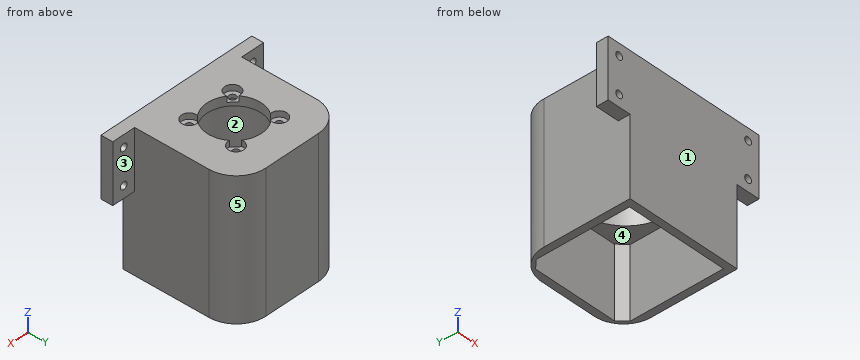
Autodesk Inventor part; units mm, degrees
ref_plane "YZ Plane" through (0, 0, 0) normal (1, 0, 0) x (0, 1, 0)
ref_plane "XZ Plane" through (0, 0, 0) normal (0, 1, 0) x (-1, 0, 0)
ref_plane "XY Plane" through (0, 0, 0) normal (0, 0, 1) x (1, 0, 0)
sketch "Sketch1" plane through (0, 0, 0) normal (0, 0, 1) x (1, 0, 0)
  line L0 (-21.5, -21.5) -> (21.5, -21.5)
  line L1 (21.5, -21.5) -> (21.5, 21.5)
  line L2 (21.5, 21.5) -> (-21.5, 21.5)
  line L3 (-21.5, 21.5) -> (-21.5, -21.5)
  line L4 (-21.5, -21.5) -> (21.5, 21.5) construction
  line L5 (21.5, -21.5) -> (-21.5, 21.5) construction
  circle A0 centre (0, 0) radius 18.5
  circle A1 centre (0, 0) radius 11.5
  circle A2 centre (0, 0) radius 14
  circle A3 centre (-9.8995, 9.8995) radius 1.5
  circle A4 centre (-9.8995, -9.8995) radius 1.5
  circle A5 centre (9.8995, -9.8995) radius 1.5
  circle A6 centre (9.8995, 9.8995) radius 1.5
  line L6 (0, 0) -> (0, 21.5)
  line L7 (-24.5, 24.5) -> (24.5, 24.5)
  line L8 (24.5, 24.5) -> (24.5, -24.5)
  line L9 (24.5, -24.5) -> (-24.5, -24.5)
  line L10 (-24.5, -24.5) -> (-24.5, 24.5)
  line L11 (-24.5, 24.5) -> (24.5, -24.5) construction
  line L12 (24.5, 24.5) -> (-24.5, -24.5) construction
  dimension "d4" = 28
  dimension "d0" = 43
  dimension "d1" = 43
  dimension "d2" = 37
  dimension "d3" = 23
  dimension "d5" = 3
  dimension "d8" = 360
  dimension "d10" = 3
  dimension "d11" = 3
extrude "Extrusion1" add sketch "Sketch1" along normal blind 5 and the other way blind 30 contours L7 L8 L9 L10
extrude "Extrusion2" add sketch "Sketch1" along normal blind 24 contours L3 L2 L1 L0
sketch "Sketch2" plane through (0, 0, 24) normal (0, 0, 1) x (1, 0, 0)
  circle A0 centre (0, 0) radius 11.5
  circle A1 centre (0, 0) radius 14
  circle A2 centre (9.8995, 9.8995) radius 1.5
  circle A3 centre (9.8995, -9.8995) radius 1.5
  circle A4 centre (-9.8995, -9.8995) radius 1.5
  circle A5 centre (-9.8995, 9.8995) radius 1.5
  circle A6 centre (0, 0) radius 18.5
  line L0 (-21.5, 21.5) -> (-21.5, -21.5)
  line L1 (-21.5, -21.5) -> (21.5, -21.5)
  line L2 (21.5, -21.5) -> (21.5, 21.5)
  line L3 (21.5, 21.5) -> (-21.5, 21.5)
  circle A7 centre (0, 0) radius 18.5
  line L4 (24.5, -24.5) -> (-24.5, -24.5)
  line L5 (24.5, 24.5) -> (24.5, -24.5)
  line L6 (-24.5, 24.5) -> (24.5, 24.5)
  line L7 (-24.5, -24.5) -> (-24.5, 24.5)
  line L8 (21.5, -21.5) -> (21.5, 21.5)
  line L9 (-21.5, -21.5) -> (21.5, -21.5)
  line L10 (-21.5, 21.5) -> (-21.5, -21.5)
  line L11 (21.5, 21.5) -> (-21.5, 21.5)
extrude "Extrusion3" add sketch "Sketch2" along normal blind 4 contours A1 A3 A4 A5 A2 | A6 | L3 L2 L1 L0
sketch "Sketch8" plane through (0, 0, 28) normal (0, 0, 1) x (1, 0, 0)
  line L0 (-24.5, -24.5) -> (24.5, -24.5)
  line L1 (24.5, -24.5) -> (24.5, 24.5)
  line L2 (24.5, 24.5) -> (-24.5, 24.5)
  line L3 (-24.5, 24.5) -> (-24.5, -24.5)
  line L4 (21.5, 21.5) -> (21.5, -21.5)
  line L5 (21.5, -21.5) -> (-21.5, -21.5)
  line L6 (-21.5, -21.5) -> (-21.5, 21.5)
  line L7 (-21.5, 21.5) -> (21.5, 21.5)
  line L8 (-21.5, 21.5) -> (-21.5, -21.5)
  line L9 (-21.5, -21.5) -> (21.5, -21.5)
  line L10 (21.5, -21.5) -> (21.5, 21.5)
  line L11 (21.5, 21.5) -> (-21.5, 21.5)
  circle A0 centre (-9.8995, 9.8995) radius 1.5
  circle A1 centre (-9.8995, -9.8995) radius 1.5
  circle A2 centre (9.8995, -9.8995) radius 1.5
  circle A3 centre (0, 0) radius 11.5
  circle A4 centre (9.8995, 9.8995) radius 1.5
extrude "Extrusion8" add sketch "Sketch8" against normal up to surface (23 mm away) contours L3 L2 L1 L0
sketch "Sketch9" plane through (-24.5, -24.5, -30) normal (0, -1, 0) x (1, 0, 0)
  line L0 (49, 0) -> (49, 58)
  line L1 (49, 58) -> (59, 58)
  line L2 (59, 58) -> (59, 33)
  line L3 (59, 33) -> (49, 33)
  line L4 (49, 33) -> (49, 58)
  line L5 (0, 58) -> (0, 0)
  line L6 (0, 58) -> (-10, 58)
  line L7 (-10, 58) -> (-10, 33)
  line L8 (-10, 33) -> (0, 33)
  line L9 (0, 33) -> (0, 58)
  line L10 (0, 58) -> (49, 58)
  circle A0 centre (54, 38) radius 1.55
  circle A1 centre (54, 53) radius 1.55
  circle A2 centre (-5, 38) radius 1.55
  circle A3 centre (-5, 53) radius 1.55
  point P0 (24.5, 30)
  point P1 (0, 33)
  point P2 (49, 33)
  dimension "d72" = 0
  dimension "d73" = 25
  dimension "d74" = 25
  dimension "d75" = 10
  dimension "d76" = 10
  dimension "d77" = 15
  dimension "d78" = 15
  dimension "d79" = 5
  dimension "d80" = 5
  dimension "d81" = 3.1
  dimension "d82" = 3.1
  dimension "d83" = 3.1
  dimension "d84" = 3.1
extrude "Extrusion9" add sketch "Sketch9" against normal blind 5
chamfer "Chamfer3" distance 3.5 angle 45 2 edges at (21.5, 21.5, -15) (-21.5, 21.5, -15)
fillet "Fillet10" radius 12.5 2 edges at (-24.5, 24.5, -1) (24.5, 24.5, -1)
sketch "Sketch10" plane through (0, 0, 28) normal (0, 0, 1) x (1, 0, 0)
  circle A0 centre (-9.8995, 9.8995) radius 1.5
  circle A1 centre (-9.8995, 9.8995) radius 3.25
  circle A2 centre (9.8995, 9.8995) radius 1.5
  circle A3 centre (9.8995, 9.8995) radius 3.25
  circle A4 centre (9.8995, -9.8995) radius 1.5
  circle A5 centre (9.8995, -9.8995) radius 3.25
  circle A6 centre (-9.8995, -9.8995) radius 1.5
  circle A7 centre (-9.8995, -9.8995) radius 3.25
  point P0 (0, 0)
  dimension "d94" = 6.5
  dimension "d95" = 6.5
  dimension "d96" = 6.5
  dimension "d97" = 6.5
extrude "Extrusion10" cut sketch "Sketch10" against normal blind 2.5 contours A0 | A1 | A2 | A3 | A4 | A5 | A6 | A7
properties part number "StepperMotorHolder"
For this review, take the finished solid that the model builds, in its own axes (mm). Face numbers are marked on the shaded views. A direction names the side the tool comes from. Round coordinates to 2 decimals unless told otherwise and drop trailing zeros. Write each loop counter-clockwise with the first axis right and the second up, starting at its lowest first coordinate (ties: lowest second). Pieces come first, ordered by that corner, then holes. Notation, with made-up numbers: (35.5, 26.25) -> (54.5, 26.25) arc R14 ccw to (54.5, 51.25) -> close; hole circle Ø1 at (29, -29). An arc over 180 degrees is marked (long way). Use one line per item in the form item = value.
1) Clearance check with flat-ended pins moving along their axes: pin 1 (3 mm diameter, centred on x = -16, y = 17.5, fed in from -Z); pin 2 (6 mm diameter, centred on y = -16, z = -13.5, fed in from -X); pin 3 (10 mm diameter, centred on y = 6, z = 20, fed in from +X). State where each tip first meets the part, or that it passes through.
Found:
pin_1 = 0
pin_2 = -24.5
pin_3 = 24.5
2) Tool access review of the marked faces 1 and 2: name each direction out of +Z, -Z, +X, -X, +Y, -Y from which nothing blocks a thin tool from reaching the whole face with its end or side.
Found:
face_1 = +Z, -Z, +X, -X, -Y
face_2 = -Z
3) To check wall thickness, follow L1, parallel to Z at x = 29.5, y = -21.9; L2, parallel to X at y = -9, z = -28; L3, parallel to Y at x = 12.5, z = -1. State the ranges of each line that lie inside material, in increasing order. Write a range as from..to.
Found:
L1 = 3..6.45, 9.55..21.45, 24.55..28
L2 = -24.5..-21.5, 21.5..24.5
L3 = -24.5..-21.5, 21.5..24.49
4) Take a section at C-C, the plane x = -29.5. Write out the cut boundary in (y, z).
Found:
outline = (-24.5, 3) -> (-19.5, 3) -> (-19.5, 6.45) -> (-24.5, 6.45) -> close; (-24.5, 9.55) -> (-19.5, 9.55) -> (-19.5, 21.45) -> (-24.5, 21.45) -> close; (-24.5, 24.55) -> (-19.5, 24.55) -> (-19.5, 28) -> (-24.5, 28) -> close
5) Take a section at B-B, the plane y = 0. Write out the cut boundary in (x, z).
Found:
outline = (-24.5, -30) -> (-21.5, -30) -> (-21.5, 0) -> (-18.5, 0) -> (-18.5, 24) -> (-11.5, 24) -> (-11.5, 28) -> (-24.5, 28) -> close; (11.5, 24) -> (18.5, 24) -> (18.5, 0) -> (21.5, 0) -> (21.5, -30) -> (24.5, -30) -> (24.5, 28) -> (11.5, 28) -> close
6) Mouldability with a two-part tool opening along X and no side actions: class the marked faces 3, 4 and 5 as +X half, -X half, draft (parallel to the pull), parting line (faces both ways), or undercut.
Found:
face_3 = draft
face_4 = undercut
face_5 = +X half
7) Take a section at A-A, the plane z = 23. Write out the cut boundary in (x, y), and give its area (3 significant figures).
Found:
outline = (-34.5, -24.5) -> (-31.05, -24.5) -> (-31.05, -19.5) -> (-34.5, -19.5) -> close; (-27.95, -24.5) -> (27.95, -24.5) -> (27.95, -19.5) -> (24.5, -19.5) -> (24.5, 12) arc R12.5 ccw to (12, 24.5) -> (-12, 24.5) arc R12.5 ccw to (-24.5, 12) -> (-24.5, -19.5) -> (-27.95, -19.5) -> close; (31.05, -24.5) -> (34.5, -24.5) -> (34.5, -19.5) -> (31.05, -19.5) -> close; hole circle Ø37 at (0, 0)
area = 1,330 mm2
